The listing builds one solid part. Answer for the finished solid, in the listing's coordinates (mm). Face numbers are marked on the shaded views. Round coordinates to 2 decimals unless told otherwise and drop trailing zeros. Write each loop counter-clockwise with the first axis right and the second up, starting at its lowest first coordinate (ties: lowest second). Pieces come first, ordered by that corner, then holes. Notation, with made-up numbers: (30.5, -19.5) - (64.5, -19.5) arc R20 cw to (64.5, 18.5) - close; hole circle Ø10 at (89, -16.75). An arc over 180 degrees is marked (long way). Answer as CSV lines item,"result". Start each with the question number.
Item 1: A cutting plane is placed at B-B on z = -0.2. Determine the outline of the cut face in (x, y).
Item 2: A cutting plane is placed at C-C on x = 0.45. Determine the outline of the cut face in (y, z).
Item 3: A cutting plane is placed at D-D on y = 8.5. Determine the outline of the cut face in (x, z).
Item 4: Straight lines are drawn through the part: line 1 along Z through (x, y) = (0.8, 9.75); line 2 along X through (y, z) = (12.5, 1.05); line 3 along Y through (x, z) = (0.45, 2.9). For each, find the intervals that lie inside material, in ascending order. Write a range as [from, to].
Item 5: Flat-ended cylindrical pins translate along their axes: pin 1 (0.5 mm diameter, centred on x = 1, y = 8, fed in from +Z); pin 2 (2 mm diameter, centred on y = 3, z = -0.5, fed in from -X); pin 3 (1 mm diameter, centred on x = 0.5, y = 4, fed in from -Z). Find the tip coordinate at first contact, or state that the pin passes through.
Item 6: For a pull along Z with two mould halves and no side action, classify the marked faces 1, 2 and 3 as pulls with the +Z half, pulls with the -Z half, needs draft (parallel to the pull), parting line crosses it, or undercut.
Item 7: A cutting plane is placed at A-A on x = -0.2. Determine the outline of the cut face in (y, z).
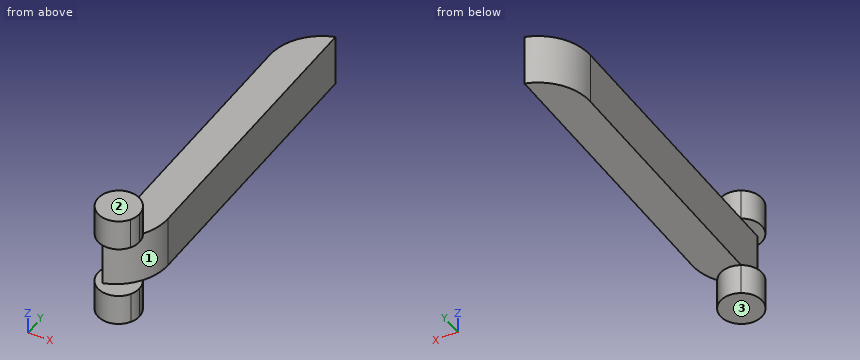
```python
from build123d import *

# Parameters (mm, degrees)
F0_W        = 16
F0_H        = 2.5
F1_DEPTH    = 1.75
F4_DEPTH    = 1.5
F5_DEPTH    = 1.5
F6_T1_DEPTH = 14.4242400177
F6_T3_DEPTH = 2.5


# Not quite as in the source:
# - a fillet or chamfer that OpenCascade refuses, or shapes differently, is made with other operations: its cross-section is extruded or revolved along the edge and cut away or added


with BuildPart() as f1:
    # F0 (on Right) → F1 (new body)
    with BuildSketch(Plane.YZ):
        with Locations((8, 1.25)):
            Rectangle(F0_W, F0_H)
    extrude(amount=F1_DEPTH)

    # F3 (on face) → F4 (join)
    with BuildSketch(Plane.XY.offset(2.5)):
        with BuildLine():
            ThreePointArc((1.3660254038, 0), (1.4659258263, 0.2411809549), (1.5, 0.5))
            ThreePointArc((1.5, 0.5), (1, 1.3660254038), (0, 1.3660254038))
            Line((0, 1.3660254038), (0, 0))
            Line((0, 0), (1.3660254038, 0))
        make_face()
        with BuildLine():
            Line((0, 0), (0, 1.3660254038))
            ThreePointArc((0, 1.3660254038), (-0.2071067812, -0.2071067812), (1.3660254038, 0))
            Line((1.3660254038, 0), (0, 0))
        make_face()
    extrude(amount=F4_DEPTH)

    # F2 (on face) → F5 (join)
    with BuildSketch(Plane(origin=(0, 0, 0), x_dir=(1, 0, 0), z_dir=(0, 0, -1))):
        with BuildLine():
            ThreePointArc((0, -1.3527675268), (1, -1.3527675268), (1.5, -0.486742123))
            ThreePointArc((1.5, -0.486742123), (1.4678702674, -0.2352920375), (1.373545709, 0))
            Line((1.373545709, 0), (0, 0))
            Line((0, 0), (0, -1.3527675268))
        make_face()
        with BuildLine():
            Line((0, 0), (1.373545709, 0))
            ThreePointArc((1.373545709, 0), (-0.2016972955, 0.2257330733), (0, -1.3527675268))
            Line((0, -1.3527675268), (0, 0))
        make_face()
    extrude(amount=F5_DEPTH)

    # F6: fillet of radius 2.5 on 2 edges, made by hand

    # F6_s2 → F6_t1 (cut)
    with BuildSketch(Plane.XY.offset(-5.9621200089)):
        with BuildLine():
            ThreePointArc((0, 13.6151519965), (0.4844355629, 15.0941719422), (1.75, 16))
            Line((1.75, 16), (0, 16))
            Line((0, 16), (0, 13.6151519965))
        make_face()
    extrude(amount=F6_T1_DEPTH, mode=Mode.SUBTRACT)

    # F6_s4 → F6_t3 (cut)
    with BuildSketch(Plane.XY):
        with BuildLine():
            ThreePointArc((0, 0), (1.2655644371, 0.9058280578), (1.75, 2.3848480035))
            Line((1.75, 2.3848480035), (1.75, 0))
            Line((1.75, 0), (0, 0))
        make_face()
    extrude(amount=F6_T3_DEPTH, mode=Mode.SUBTRACT)


solid = f1.part
```
Geometry says:
1,outline,"circle Ø2 at (0.5, 0.49)"
2,outline,"(-0.51, -1.5) - (1.49, -1.5) - (1.49, 0) - (15.05, 0) - (15.05, 2.5) - (1.5, 2.5) - (1.5, 4) - (-0.5, 4) - (-0.5, 2.5) - (0.19, 2.5) - (0.19, 0) - (-0.51, 0) - close"
3,outline,"(0, 0) - (1.75, 0) - (1.75, 2.5) - (0, 2.5) - close"
4,line 1,"z = [0, 2.5]"
4,line 2,"x = [0, 1.75]"
4,line 3,"y = [-0.5, 1.5]"
5,pin 1,"stops at z = 2.5"
5,pin 2,"stops at x = 0"
5,pin 3,"stops at z = 0"
6,face 1,"undercut"
6,face 2,"pulls with the +Z half"
6,face 3,"pulls with the -Z half"
7,outline,"(-0.23, -1.5) - (1.2, -1.5) - (1.2, 0) - (-0.23, 0) - close; (-0.21, 2.5) - (1.21, 2.5) - (1.21, 4) - (-0.21, 4) - close"
